Print and shaded views of the part. All mm, measured from the part's lowest x, y and z. Give positions to 0.01 mm unless a question says otherwise; leave off trailing zeros. Write each loop counter-clockwise with the first axis right and the second up, starting at its lowest first coordinate (ties: lowest second). Pieces come first, ordered by that corner, then holes. Notation, with made-up numbers: (-21, 89) -> (-4, 89) arc R34 ccw to (-4, 119) -> close; hole circle Ø4 at (38.5, 80.5). An arc over 180 degrees is marked (long way). Put each result on its own line as item: value.
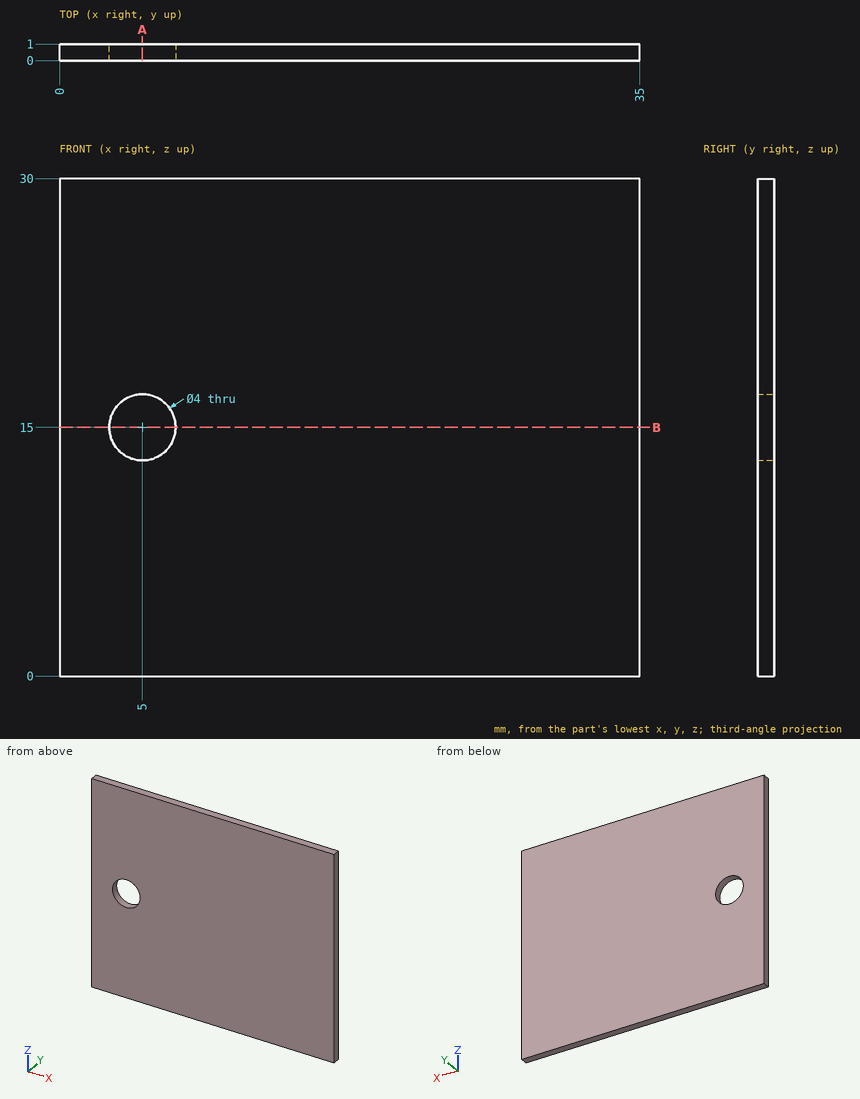
1) Wall check: L1, parallel to Z at x = 5, y = 0.4; L2, parallel to X at y = 0.6, z = 15; L3, parallel to X at y = 0.55, z = 15.5. Give the ranges that are in metal, low to high.
Filled sheet:
L1: 0 to 13, 17 to 30
L2: 0 to 3, 7 to 35
L3: 0 to 3.06, 6.94 to 35
2) Slice it at A-A (x = 5). Write the cut outline in (y, z), plus the area to 3 significant figures.
Filled sheet:
outline: (0, 0) -> (1, 0) -> (1, 13) -> (0, 13) -> close; (0, 17) -> (1, 17) -> (1, 30) -> (0, 30) -> close
area: 26.0 mm2
3) Slice it at B-B (z = 15). Write the cut outline in (x, y).
Filled sheet:
outline: (0, 0) -> (3, 0) -> (3, 1) -> (0, 1) -> close; (7, 0) -> (35, 0) -> (35, 1) -> (7, 1) -> close
